Could you check a few things on this model? Use its own coordinates, in mm. Coordinates: 2 decimals unless noted, no trailing zeros. Loops run counter-clockwise (first coordinate to the right, second up) from the corner with the lowest first, then second, coordinate; pieces in that order, holes last.
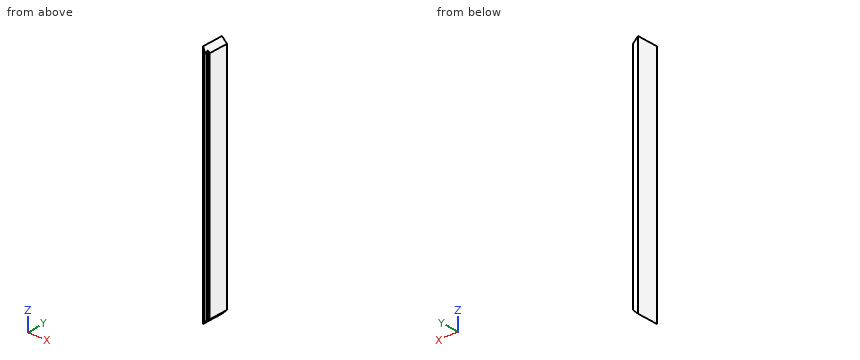
from build123d import *

# Parameters (mm, degrees)
F0_W     = 88.9
F0_H     = 914.4
F1_DEPTH = 19.05
F2_W     = 6.35
F2_H     = 914.4
F3_DEPTH = 6.35
F4_SIZE2 = 5.08
F4_SIZE  = 10.16
F6_DEPTH = 88.901


with BuildPart() as f1:
    # F0 (on Right) → F1 (new body)
    with BuildSketch(Plane.YZ):
        with Locations((44.45, 457.2)):
            Rectangle(F0_W, F0_H)
    extrude(amount=F1_DEPTH)

    # F2 (on face) → F3 (cut)
    with BuildSketch(Plane.YZ.offset(19.05)):
        with Locations((9.525, 457.2)):
            Rectangle(F2_W, F2_H)
    extrude(amount=-F3_DEPTH, mode=Mode.SUBTRACT)

    # F4
    f4_edges = [f1.edges().sort_by_distance(p)[0] for p in [
        (0, 0, 457.2),
    ]]
    chamfer(f4_edges, length=F4_SIZE, length2=F4_SIZE2)

    # F5 (on face) → F6 (cut, through all)
    with BuildSketch(Plane(origin=(0, 88.9, 0), x_dir=(-1, 0, 0), z_dir=(0, 1, 0))):
        Polygon((-19.05, 895.35), (0, 914.4), (-19.05, 914.4), align=None)
        Polygon((-19.05, 0), (0, 0), (-19.05, 19.05), align=None)
    extrude(amount=-F6_DEPTH, mode=Mode.SUBTRACT)


solid = f1.part
(1) I need wall thicknesses on probe 1 along Y at (x, z) = (14.5, 137); probe 2 along Z at (x, y) = (6.5, 63.5); probe 3 along Y at (x, z) = (9.5, 779). Which ranges of each line are inside material? Lowest first, please.
Answers:
probe 1: y = 0 to 6.35, 12.7 to 88.9
probe 2: z = 6.5 to 907.9
probe 3: y = 0.33 to 88.9
(2) Imagine slicing it at A-A, the plane x = 16. Write out the boundary of the cut face in (y, z), and give its area (3 significant figures).
Answers:
outline: (0, 16) - (6.35, 16) - (6.35, 898.4) - (0, 898.4) - close; (12.7, 16) - (88.9, 16) - (88.9, 898.4) - (12.7, 898.4) - close
area: 72,800 mm2
(3) Imagine slicing it at C-C, the plane y = 41.5. Write out the boundary of the cut face in (x, z).
Answers:
outline: (0, 0) - (19.05, 19.05) - (19.05, 895.35) - (0, 914.4) - close
(4) Imagine slicing it at B-B, the plane z = 209. Write out the boundary of the cut face in (x, y).
Answers:
outline: (0, 5.08) - (10.16, 0) - (19.05, 0) - (19.05, 6.35) - (12.7, 6.35) - (12.7, 12.7) - (19.05, 12.7) - (19.05, 88.9) - (0, 88.9) - close
(5) For pin 1 (2 mm diameter, centred on x = 2, z = 209, fed in from -Y); pin 2 (10 mm diameter, centred on x = 14, y = 20, fed in from -Z); pin 3 (6 mm diameter, centred on x = 10.5, y = 21.5, fed in from +Z), each with a flat end and sliding along its axis, tell me the tip position at first contact or that it passes through.
Answers:
pin 1: stops at y = 3.58
pin 2: stops at z = 9
pin 3: stops at z = 906.9
